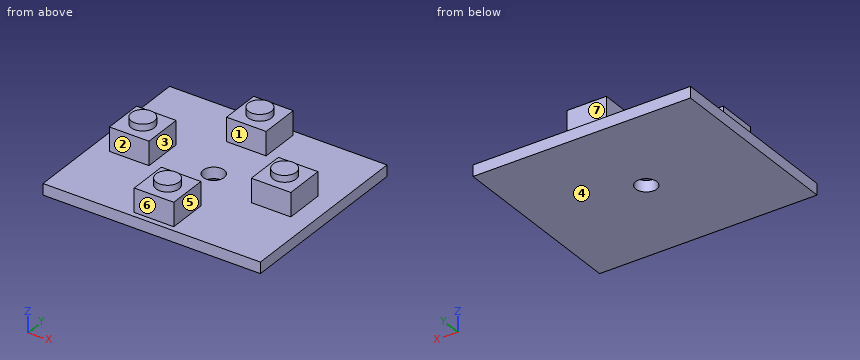
```python
from build123d import *

# Parameters (mm, degrees)
CYLINDER001_R     = 1.75
CYLINDER001_DEPTH = 1
BOX002_W          = 6
BOX002_H          = 6
BOX002_DEPTH      = 3.6
CYLINDER002_R     = 1.75
CYLINDER002_DEPTH = 1
BOX003_W          = 6
BOX003_H          = 6
BOX003_DEPTH      = 3.6
CYLINDER003_R     = 1.75
CYLINDER003_DEPTH = 1
BOX004_W          = 6
BOX004_H          = 6
BOX004_DEPTH      = 3.6
CYLINDER004_R     = 1.588
CYLINDER004_DEPTH = 2
BOX001_W          = 33
BOX001_H          = 28
BOX001_DEPTH      = 1.7
CYLINDER_R        = 1.75
CYLINDER_DEPTH    = 1
BOX_W             = 6
BOX_H             = 6
BOX_DEPTH         = 3.6


with BuildPart() as obj1:
    # Cylinder001 → Cylinder001 (new body)
    with BuildSketch(Plane(origin=(3, 3, 3.6), x_dir=(1, 0, 0), z_dir=(0, 0, 1))):
        Circle(CYLINDER001_R)
    extrude(amount=CYLINDER001_DEPTH)


with BuildPart() as obj2:
    # Box002 → Box002 (new body)
    with BuildSketch(Plane.XY):
        with Locations((3, 3)):
            Rectangle(BOX002_W, BOX002_H)
    extrude(amount=BOX002_DEPTH)

    # Fusion011: union obj1
    add(obj1.part)


with BuildPart() as obj2_1:
    # Fusion011 placement: moved
    add(obj2.part.moved(Location((24.07, 11, 1.7))))


with BuildPart() as obj3:
    # Cylinder002 → Cylinder002 (new body)
    with BuildSketch(Plane(origin=(3, 3, 3.6), x_dir=(1, 0, 0), z_dir=(0, 0, 1))):
        Circle(CYLINDER002_R)
    extrude(amount=CYLINDER002_DEPTH)


with BuildPart() as obj4:
    # Box003 → Box003 (new body)
    with BuildSketch(Plane.XY):
        with Locations((3, 3)):
            Rectangle(BOX003_W, BOX003_H)
    extrude(amount=BOX003_DEPTH)

    # Fusion010: union obj3
    add(obj3.part)


with BuildPart() as obj4_1:
    # Fusion010 placement: moved
    add(obj4.part.moved(Location((13.31, 21.21, 1.7))))


with BuildPart() as obj5:
    # Cylinder003 → Cylinder003 (new body)
    with BuildSketch(Plane(origin=(3, 3, 3.6), x_dir=(1, 0, 0), z_dir=(0, 0, 1))):
        Circle(CYLINDER003_R)
    extrude(amount=CYLINDER003_DEPTH)


with BuildPart() as obj6:
    # Box004 → Box004 (new body)
    with BuildSketch(Plane.XY):
        with Locations((3, 3)):
            Rectangle(BOX004_W, BOX004_H)
    extrude(amount=BOX004_DEPTH)

    # Fusion009: union obj5
    add(obj5.part)


with BuildPart() as obj6_1:
    # Fusion009 placement: moved
    add(obj6.part.moved(Location((13.31, 0.787, 1.7))))


with BuildPart() as obj7:
    # Cylinder004 → Cylinder004 (new body)
    with BuildSketch(Plane(origin=(16.31, 14, 0), x_dir=(1, 0, 0), z_dir=(0, 0, 1))):
        Circle(CYLINDER004_R)
    extrude(amount=CYLINDER004_DEPTH)


with BuildPart() as cut006:
    # Box001 → Box001 (new body)
    with BuildSketch(Plane.XY):
        with Locations((16.5, 14)):
            Rectangle(BOX001_W, BOX001_H)
    extrude(amount=BOX001_DEPTH)

    # Cut006: cut obj7
    add(obj7.part, mode=Mode.SUBTRACT)


with BuildPart() as obj8:
    # Cylinder → Cylinder (new body)
    with BuildSketch(Plane(origin=(3, 3, 3.6), x_dir=(1, 0, 0), z_dir=(0, 0, 1))):
        Circle(CYLINDER_R)
    extrude(amount=CYLINDER_DEPTH)


with BuildPart() as main_buttons_pcb:
    # Box → Box (new body)
    with BuildSketch(Plane.XY):
        with Locations((3, 3)):
            Rectangle(BOX_W, BOX_H)
    extrude(amount=BOX_DEPTH)

    # Fusion012: union obj8
    add(obj8.part)


with BuildPart() as main_buttons_pcb_1:
    # Fusion012 placement: moved
    add(main_buttons_pcb.part.moved(Location((2.54, 11, 1.7))))

    # Fusion008: union obj2, obj4, obj6, Cut006
    add(obj2_1.part)
    add(obj4_1.part)
    add(obj6_1.part)
    add(cut006.part)


with BuildPart() as main_buttons_pcb_2:
    # Fusion008 placement: moved
    add(main_buttons_pcb_1.part.moved(Location((86, 0, 0))))


solid = main_buttons_pcb_2.part
```
CAD build for the part. Positions are in the model's coordinates, mm. Face numbers are marked on the shaded views. A direction names the side the tool comes from. Coordinates: 2 decimals unless noted, no trailing zeros. Order: outer loops, then holes, each group sorted by start corner. A loop starts at its lowest first (then second) coordinate and runs counter-clockwise, first axis right, second up.
(1) Pin check, flat tips, straight feed: pin 1 Ø1.8 at (x, z) = (93, 4) entering from +Y; pin 2 Ø1.1 at (x, z) = (114, 4) entering from -Y; pin 3 Ø1 at (y, z) = (18.5, 4) entering from -X; pin 4 Ø1.1 at (y, z) = (24.5, 4.5) entering from +X. Stop position of each tip, or through.
Solution:
pin 1: stops at y = 17
pin 2: stops at y = 11
pin 3: passes through
pin 4: stops at x = 105.31
(2) Saw through at A-A, the plane y = 14. Write the cut outline in (x, z), and give its area (3 significant figures).
Solution:
outline: (86, 0) - (100.72, 0) - (100.72, 1.7) - (94.54, 1.7) - (94.54, 5.3) - (93.29, 5.3) - (93.29, 6.3) - (89.79, 6.3) - (89.79, 5.3) - (88.54, 5.3) - (88.54, 1.7) - (86, 1.7) - close; (103.9, 0) - (119, 0) - (119, 1.7) - (116.07, 1.7) - (116.07, 5.3) - (114.82, 5.3) - (114.82, 6.3) - (111.32, 6.3) - (111.32, 5.3) - (110.07, 5.3) - (110.07, 1.7) - (103.9, 1.7) - close
area: 101 mm2
(3) Drill centre lines: L1, parallel to X at y = 14, z = 0.6; L2, parallel to Y at x = 102.31, z = 1.1; L3, parallel to Y at x = 104.5, z = 4.5. Where is each one in solid material? Low to high.
Solution:
L1: x = 86 to 100.72, 103.9 to 119
L2: y = 0 to 12.41, 15.59 to 28
L3: y = 0.79 to 6.79, 21.21 to 27.21
(4) Saw through at B-B, the plane z = 4.5. Write the cut outline in (x, y).
Solution:
outline: (88.54, 11) - (94.54, 11) - (94.54, 17) - (88.54, 17) - close; (99.31, 0.79) - (105.31, 0.79) - (105.31, 6.79) - (99.31, 6.79) - close; (99.31, 21.21) - (105.31, 21.21) - (105.31, 27.21) - (99.31, 27.21) - close; (110.07, 11) - (116.07, 11) - (116.07, 17) - (110.07, 17) - close
(5) Mould opens along Y. For the marked faces 1, 2 and 3 say: released by +Y, released by -Y, zero draft, split by the parting line, or undercut.
Solution:
face 1: undercut
face 2: released by -Y
face 3: zero draft
(6) Saw through at C-C, the plane x = 102.31. Write the cut outline in (y, z).
Solution:
outline: (0, 0) - (12.41, 0) - (12.41, 1.7) - (6.79, 1.7) - (6.79, 5.3) - (5.54, 5.3) - (5.54, 6.3) - (2.04, 6.3) - (2.04, 5.3) - (0.79, 5.3) - (0.79, 1.7) - (0, 1.7) - close; (15.59, 0) - (28, 0) - (28, 1.7) - (27.21, 1.7) - (27.21, 5.3) - (25.96, 5.3) - (25.96, 6.3) - (22.46, 6.3) - (22.46, 5.3) - (21.21, 5.3) - (21.21, 1.7) - (15.59, 1.7) - close
(7) Saw through at D-D, the plane y = 24.21. Write the cut outline in (x, z).
Solution:
outline: (86, 0) - (119, 0) - (119, 1.7) - (105.31, 1.7) - (105.31, 5.3) - (104.06, 5.3) - (104.06, 6.3) - (100.56, 6.3) - (100.56, 5.3) - (99.31, 5.3) - (99.31, 1.7) - (86, 1.7) - close
(8) Which spindle directions (+Z, -Z, +X, -X, +Y, -Y) get a long thin tool onto all of the face, cutting with end or side? Do the marked faces 4, 5, 6 and 7. Say none if no direction does.
Solution:
face 4: -Z, +X, -X, +Y, -Y
face 5: +Z, +X, +Y, -Y
face 6: +Z, +X, -X, -Y
face 7: +Z, +X, -X, +Y
